Here's how the part is built. I have some questions about the finished solid (model axes, mm). Round coordinates to 2 decimals unless told otherwise and drop trailing zeros. One line per question, with ' | ' between items. Start each with the question number.
(1) If I drill on L1, parallel to X at y = -30, z = -107; L2, parallel to Z at x = 1, y = -19; L3, parallel to Y at x = 1.25, z = -552.45 (3 decimals), over which ranges is the centre line in solid material (lowest first)?
(2) Thinking about a two-plate mould opening in X: for faces 1 (the flat face through (1205.33, -12.52, -289.75)), 2 (the flat face through (0, -19, -282)), 3 (the flat face through (601, -38.1, -282)), which applies, pulls with the +X half, pulls with the -X half, needs draft (parallel to the pull), parting line crosses it, or undercut?
(3) Will these pins go through, and if not, where does the flat tip stop? pin 1 (2.5 mm diameter, centred on x = 1167.5, z = -106.5, fed in from -Y); pin 2 (12 mm diameter, centred on y = -13, z = -414.5, fed in from +X); pin 3 (10 mm diameter, centred on y = -19.05, z = -552.45, fed in from +X).
from build123d import *

# Parameters (mm, degrees)
F1_DEPTH = 38.1
F3_D     = 6.35
F3_DEPTH = 1.524
F3_TIP   = 1.9077324654
F4_SIZE2 = 25.4
F4_SIZE  = 25.4
F6_DEPTH = 12.7
F7_R     = 3.9751
F8_DEPTH = 12.7


with BuildPart() as f1:
    # F0 (on Front) → F1 (new body)
    with BuildSketch(Plane.XZ):
        Polygon((0, -6.35), (0, -571.5), (1218.2094, -571.5), (1218.2094, -6.35), (1218.2094, 0), (0, 0), align=None)
    extrude(amount=F1_DEPTH)

    # F3
    with Locations(Plane(origin=(0, 0, 0), x_dir=(0, -1, 0), z_dir=(-1, 0, 0))):
        with Locations((19.05, -552.45), (19.05, -590.55)):
            Hole(F3_D / 2, depth=F3_DEPTH)
            with Locations((0, 0, -(F3_DEPTH + F3_TIP / 2))):  # 118° drill point
                Cone(0, F3_D / 2, F3_TIP, mode=Mode.SUBTRACT)

    # F4
    f4_edges = [f1.edges().sort_by_distance(p)[0] for p in [
        (1218.2094, 0, -285.75),
    ]]
    chamfer(f4_edges, length=F4_SIZE, length2=F4_SIZE2)

    # F5 (on face) → F6 (cut)
    with BuildSketch(Plane(origin=(596.4047, 596.4047, 0), x_dir=(-0.7071067812, 0.7071067812, 0), z_dir=(0.7071067812, 0.7071067812, 0))):
        with BuildLine():
            ThreePointArc((-864.5791276452, -561.975), (-863.6491916755, -564.2200640303), (-861.4041276452, -565.15))
            Line((-861.4041276452, -565.15), (-861.4041276452, -561.975))
            Line((-861.4041276452, -561.975), (-864.5791276452, -561.975))
        make_face()
        with BuildLine():
            ThreePointArc((-861.4041276452, -6.35), (-864.5791276452, -9.525), (-861.4041276452, -12.7))
            Line((-861.4041276452, -12.7), (-861.4041276452, -6.35))
        make_face()
        with BuildLine():
            Line((-861.4041276452, -6.35), (-861.4041276452, -12.7))
            ThreePointArc((-861.4041276452, -12.7), (-859.1590636149, -11.7700640303), (-858.2291276452, -9.525))
            ThreePointArc((-858.2291276452, -9.525), (-859.1590636149, -7.2799359697), (-861.4041276452, -6.35))
        make_face()
        with BuildLine():
            ThreePointArc((-861.4041276452, -69.85), (-864.5791276452, -73.025), (-861.4041276452, -76.2))
            Line((-861.4041276452, -76.2), (-861.4041276452, -69.85))
        make_face()
        with BuildLine():
            Line((-861.4041276452, -69.85), (-861.4041276452, -76.2))
            ThreePointArc((-861.4041276452, -76.2), (-859.1590636149, -75.2700640303), (-858.2291276452, -73.025))
            ThreePointArc((-858.2291276452, -73.025), (-859.1590636149, -70.7799359697), (-861.4041276452, -69.85))
        make_face()
        with BuildLine():
            ThreePointArc((-861.4041276452, -495.3), (-864.5791276452, -498.475), (-861.4041276452, -501.65))
            Line((-861.4041276452, -501.65), (-861.4041276452, -498.475))
            Line((-861.4041276452, -498.475), (-861.4041276452, -495.3))
        make_face()
        with BuildLine():
            Line((-861.4041276452, -498.475), (-861.4041276452, -501.65))
            ThreePointArc((-861.4041276452, -501.65), (-859.1590636149, -500.7200640303), (-858.2291276452, -498.475))
            ThreePointArc((-858.2291276452, -498.475), (-859.1590636149, -496.2299359697), (-861.4041276452, -495.3))
            Line((-861.4041276452, -495.3), (-861.4041276452, -498.475))
        make_face()
        with BuildLine():
            Line((-861.4041276452, -561.975), (-861.4041276452, -565.15))
            ThreePointArc((-861.4041276452, -565.15), (-859.1590636149, -564.2200640303), (-858.2291276452, -561.975))
            ThreePointArc((-858.2291276452, -561.975), (-859.1590636149, -559.7299359697), (-861.4041276452, -558.8))
            Line((-861.4041276452, -558.8), (-861.4041276452, -561.975))
        make_face()
        with BuildLine():
            Line((-864.5791276452, -561.975), (-861.4041276452, -561.975))
            Line((-861.4041276452, -561.975), (-861.4041276452, -558.8))
            ThreePointArc((-861.4041276452, -558.8), (-863.6491916755, -559.7299359697), (-864.5791276452, -561.975))
        make_face()
    extrude(amount=-F6_DEPTH, mode=Mode.SUBTRACT)

    # F7 (on face) → F8 (cut)
    with BuildSketch(Plane.XZ.offset(38.1)):
        with BuildLine():
            ThreePointArc((1167.4094, -103.9749), (1164.5985798341, -110.7608201659), (1171.3845, -107.95))
            ThreePointArc((1171.3845, -107.95), (1170.2202201659, -105.1391798341), (1167.4094, -103.9749))
        make_face()
        with Locations((1167.4094, -463.55)):
            Circle(F7_R)
    extrude(amount=-F8_DEPTH, mode=Mode.SUBTRACT)


solid = f1.part
Check sheet entries:
1) L1: 0 to 1163.55, 1171.27 to 1218.21 | L2: -571.5 to -555.62, -549.28 to 0 | L3: -38.1 to -22.225, -15.875 to 0
2) face 1: pulls with the +X half | face 2: pulls with the -X half | face 3: needs draft
3) pin 1: y = -25.4 | pin 2: x = 1211.81 | pin 3: x = 1216.86
